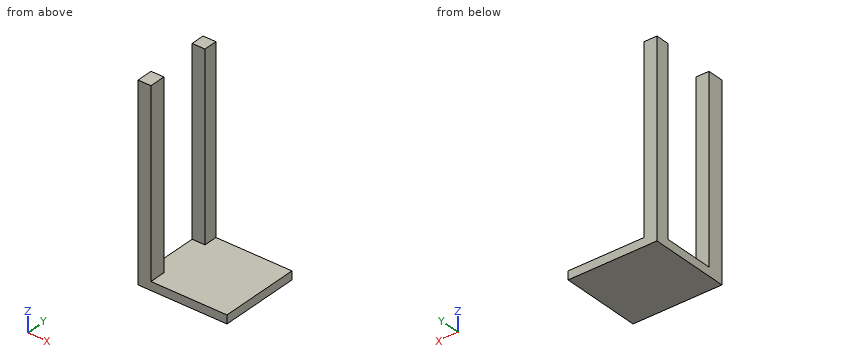
```python
from build123d import *

# Parameters (mm, degrees)
F0_W     = 16.4634734392
F0_H     = 13.1345540285
F0_H_2   = 62.0689839125
F0_W_2   = 13.7195661664
F0_W_3   = 70.2442079782
F0_H_3   = 15.9291923046
F1_DEPTH = 9.5300190151
F2_W     = 14.5427659154
F2_H     = 15.3316706419
F2_H_2   = 18.1263536215
F3_DEPTH = 205.7239394635


# Not quite as in the source:
# - the program builds the solid bodies; features that only make, move or delete a surface that nothing else refers to are left out


with BuildPart() as f1:
    # F0 (on Top) → F1 (new body)
    with BuildSketch(Plane.XY):
        with Locations((49.1160675883, 30.5517539382)):
            Rectangle(F0_W, F0_H)
        with Locations((49.1160675883, -7.0500150323)):
            Rectangle(F0_W, F0_H_2)
        with Locations((-36.2196601927, 30.5517539382)):
            Rectangle(F0_W_2, F0_H)
        with Locations((5.7622268796, 30.5517539382)):
            Rectangle(F0_W_3, F0_H)
        with Locations((-36.2196601927, -7.0500150323)):
            Rectangle(F0_W_2, F0_H_2)
        with Locations((-36.2196601927, -46.0491031408)):
            Rectangle(F0_W_2, F0_H_3)
        with Locations((5.7622268796, -46.0491031408)):
            Rectangle(F0_W_3, F0_H_3)
        with Locations((49.1160675883, -46.0491031408)):
            Rectangle(F0_W, F0_H_3)
        with Locations((5.7622268796, -7.0500150323)):
            Rectangle(F0_W_3, F0_H_2)
    extrude(amount=F1_DEPTH)

    # F2 (on face) → F3 (join)
    with BuildSketch(Plane.XY.offset(9.5300190151)):
        with Locations((-35.8080603182, 29.4531956315)):
            Rectangle(F2_W, F2_H)
        with Locations((-35.8080603182, -44.9505224824)):
            Rectangle(F2_W, F2_H_2)
    extrude(amount=F3_DEPTH)


solid = f1.part
```
Here's how the part is built. I have some questions about the finished solid (model axes, mm). Give positions to 0.01 mm unless a question says otherwise; leave off trailing zeros. Write each loop counter-clockwise with the first axis right and the second up, starting at its lowest first coordinate (ties: lowest second). Pieces come first, ordered by that corner, then holes. Notation, with made-up numbers: (5.25, -38.5) -> (24.25, -38.5) arc R12 ccw to (24.25, -24.5) -> close; hole circle Ø7 at (87.5, 53.5). An arc over 180 degrees is marked (long way). Write each question's results on one line, items separated by ' | '.
Item 1: Suppose I cut it at D-D on y = -33. Write out the boundary of the cut face in (x, z), plus the area to 3 significant figures.
Output:
outline: (-43.08, 0) -> (57.35, 0) -> (57.35, 9.53) -> (-43.08, 9.53) -> close | area: 957 mm^2
Item 2: Suppose I cut it at C-C on x = 0.5. Write out the boundary of the cut face in (y, z).
Output:
outline: (-54.01, 0) -> (37.12, 0) -> (37.12, 9.53) -> (-54.01, 9.53) -> close
Item 3: Suppose I cut it at A-A on z = 141. Write out the boundary of the cut face in (x, y), plus the area to 3 significant figures.
Output:
outline: (-43.08, -54.01) -> (-28.54, -54.01) -> (-28.54, -35.89) -> (-43.08, -35.89) -> close; (-43.08, 21.79) -> (-28.54, 21.79) -> (-28.54, 37.12) -> (-43.08, 37.12) -> close | area: 487 mm^2
Item 4: Suppose I cut it at B-B on y = 28. Write out the boundary of the cut face in (x, z), plus the area to 3 significant figures.
Output:
outline: (-43.08, 0) -> (57.35, 0) -> (57.35, 9.53) -> (-28.54, 9.53) -> (-28.54, 215.25) -> (-43.08, 215.25) -> close | area: 3,950 mm^2
Item 5: If I drill on L1, parallel to Y at x = -31, z = 53; L2, parallel to Z at x = -0.5, y = -10.5, over which ranges is the centre line in solid material (lowest first)?
Output:
L1: y = -54.01 to -35.89, 21.79 to 37.12 | L2: z = 0 to 9.53
Item 6: For pin 1 Ø8 at (x, y) = (16.5, -13) entering from +Z; pin 2 Ø12.5 at (y, z) = (33, 95.5) entering from +X, each with a flat end and sliding along its axis, tell me the tip position at first contact or that it passes through.
Output:
pin 1: stops at z = 9.53 | pin 2: stops at x = -28.54
